Could you check a few things on this model? Use its own coordinates, in mm. Round coordinates to 2 decimals unless told otherwise and drop trailing zeros. Loops run counter-clockwise (first coordinate to the right, second up) from the corner with the lowest first, then second, coordinate; pieces in that order, holes last. Notation, with made-up numbers: (2, 55.5) -> (58, 55.5) arc R8 ccw to (58, 63.5) -> close; hole circle Ø10 at (-11, 59). An arc over 180 degrees is marked (long way). One line per item, written item: value.
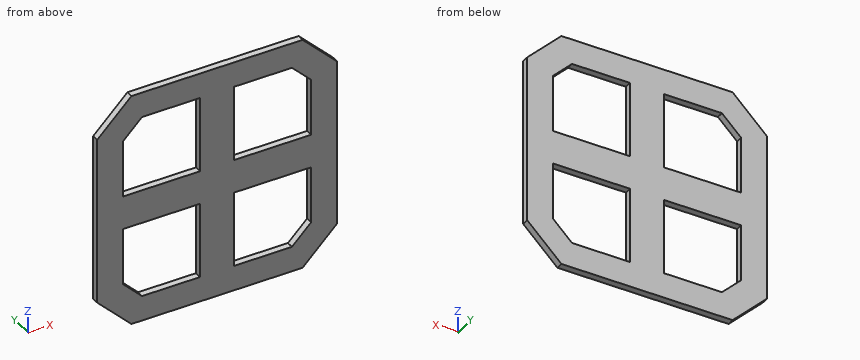
from build123d import *

# Parameters (mm, degrees)
SKETCH2_W           = 70
SKETCH2_H           = 70
BOSS_EXTRUDE1_DEPTH = 2
CUT_EXTRUDE1_DEPTH  = 2
CIRPATTERN1_COUNT   = 4


with BuildPart() as part:
    # Sketch2 → Boss-Extrude1 (new body)
    with BuildSketch(Plane(origin=(0, 0, 0), x_dir=(1, 0, 0), z_dir=(0, 1, 0))):
        Rectangle(SKETCH2_W, SKETCH2_H)
    extrude(amount=BOSS_EXTRUDE1_DEPTH)

    # Sketch4 → Cut-Extrude1 (cut)
    with BuildSketch(Plane.XZ):
        Polygon((25, 35), (35, 25), (35, 35), align=None)
        Polygon((21.893398282, 27.5), (27.5, 21.893398282), (27.5, 5), (5, 5), (5, 27.5), align=None)
    cut_extrude1 = extrude(amount=-CUT_EXTRUDE1_DEPTH, mode=Mode.SUBTRACT)

    # CirPattern1: Cut-Extrude1 ×4 about axis
    cirpattern1_axis = Axis((0, 0, 0), (0, 1, 0))
    for i in range(1, CIRPATTERN1_COUNT):
        add(cut_extrude1.rotate(cirpattern1_axis, i * 360 / CIRPATTERN1_COUNT), mode=Mode.SUBTRACT)


solid = part.part
(1) I'm going to push a flat-ended pin straight in: pin 1 Ø12 at (x, z) = (-20, 17) entering from +Y. Where does the tip first touch, or does it pass through?
Recorded:
pin 1: through
(2) If we section it at A-A, the plane z = -14: Please give me the cut outline in (x, y).
Recorded:
outline: (-35, 0) -> (-27.5, 0) -> (-27.5, 2) -> (-35, 2) -> close; (-5, 0) -> (5, 0) -> (5, 2) -> (-5, 2) -> close; (27.5, 0) -> (35, 0) -> (35, 2) -> (27.5, 2) -> close
(3) If I drill on L1, parallel to Z at x = 9.5, y = 0.55; L2, parallel to X at y = 1, z = -24, over which ranges is the centre line in solid material (lowest first)?
Recorded:
L1: -35 to -27.5, -5 to 5, 27.5 to 35
L2: -35 to -25.39, -5 to 5, 25.39 to 35
(4) If we section it at D-D, the plane z = 31.5: Please give me the cut outline in (x, y).
Recorded:
outline: (-28.5, 0) -> (28.5, 0) -> (28.5, 2) -> (-28.5, 2) -> close
(5) If we section it at B-B, the plane x = -16.5: Please give me the cut outline in (y, z).
Recorded:
outline: (0, -35) -> (2, -35) -> (2, -27.5) -> (0, -27.5) -> close; (0, -5) -> (2, -5) -> (2, 5) -> (0, 5) -> close; (0, 27.5) -> (2, 27.5) -> (2, 35) -> (0, 35) -> close
(6) If we section it at C-C, the plane y = 1.2: Please give me the cut outline in (x, z).
Recorded:
outline: (-35, -25) -> (-25, -35) -> (25, -35) -> (35, -25) -> (35, 25) -> (25, 35) -> (-25, 35) -> (-35, 25) -> close; hole (-27.5, -21.89) -> (-21.89, -27.5) -> (-5, -27.5) -> (-5, -5) -> (-27.5, -5) -> close; hole (-27.5, 5) -> (-5, 5) -> (-5, 27.5) -> (-21.89, 27.5) -> (-27.5, 21.89) -> close; hole (5, -27.5) -> (21.89, -27.5) -> (27.5, -21.89) -> (27.5, -5) -> (5, -5) -> close; hole (5, 5) -> (27.5, 5) -> (27.5, 21.89) -> (21.89, 27.5) -> (5, 27.5) -> close
